```python
from build123d import *

# Parameters (mm, degrees)
F1_DEPTH = 295.5
F3_DEPTH = 50
F5_D     = 12.5


# Not quite as in the source:
# - a pattern or mirror of a feature is missing from the dataset's text; its kind, count and spacing are read off the source's solid


with BuildPart() as f1:
    # F0 (on Right) → F1 (new body, symmetric)
    with BuildSketch(Plane.YZ):
        Polygon((0, 6), (0, 0), (50, 0), (50, 50), (44, 50), (44, 6), align=None)
    extrude(amount=F1_DEPTH, both=True)

    # F2 (on face) → F3 (join)
    with BuildSketch(Plane(origin=(0, 50, 0), x_dir=(-1, 0, 0), z_dir=(0, 1, 0))):
        Polygon((-301.5, 0), (-295.5, 0), (-295.5, 50), (-345.5, 50), (-345.5, 44), (-301.5, 44), align=None)
    f3 = extrude(amount=-F3_DEPTH)

    # F3_copies: F3 across plane
    add(f3.mirror(Plane(origin=(0, 0, 0), x_dir=(0, 0, -1), z_dir=(-1, 0, 0))))

    # F5 (through all)
    with Locations(Plane.XY.offset(50)):
        with Locations((318, 37.5), (318, 12.5)):
            f5 = Hole(F5_D / 2)

    # F5_copies: F5 across plane
    add(f5.mirror(Plane(origin=(0, 0, 0), x_dir=(0, 0, -1), z_dir=(-1, 0, 0))), mode=Mode.SUBTRACT)


solid = f1.part
```
Geometry: final body of the model. Coordinates: model frame, mm. A direction names the side the tool comes from. Round coordinates to 2 decimals unless told otherwise and drop trailing zeros. Write each loop counter-clockwise with the first axis right and the second up, starting at its lowest first coordinate (ties: lowest second). Pieces come first, ordered by that corner, then holes. Notation, with made-up numbers: M 47.25,-0.75 L 86.25,-0.75 A21 cw 86.25,38.25 Z; hole C 55,8.25 d9. An arc over 180 degrees is marked long. Answer in a Markdown table with one row per item. Add a question column.
(1) Cut plane D-D, the plane x = 219. Return the cut outline in (y, z).
(2) Cut plane A-A, the plane x = -318. Return the cut outline in (y, z).
(3) Cut plane C-C, the plane z = 32. Return the cut outline in (x, y), then the cut area to 3 significant figures.
(4) Ray query, L1, parallel to Y at x = 318, z = 46; L2, parallel to X at y = 12, z = 47; L3, parallel to X at y = 14, z = 7.5. Return the intervals inside material, ascending.
(5) Cut plane B-B, the plane y = 37.5. Return the cut outline in (x, z), then the cut area to 3 significant figures.
(6) Draft query along X for faces 1 (the face through (324.244, 12.775, 46.958)), 2 (the face through (-4, 25, 0)), 3 (the face through (-301.5, 25, 22)), 4 (the face through (-324.244, 37.775, 46.958)). Return one class per face: pulls with the +X half, pulls with the -X half, needs draft (parallel to the pull), parting line crosses it, or undercut.
(7) Reachability of faces 5 (the face through (-2, 0, 5)), 6 (the face through (295.5, 22, 28)), 7 (the face through (-324, 25, 44)), 8 (the face through (301.5, 25, 22)), 9 (the face through (2, 45, 50)) from +Z, -Z, +X, -X, +Y, -Y: full face, straight path, thin tool, end or side. Return the list, or none.
(8) Contact query for flat-ended pins moving along their axis: pin 1 (4 mm diameter, centred on y = 33, z = 34.5, fed in from -X); pin 2 (12 mm diameter, centred on y = 10.5, z = 22.5, fed in from +X); pin 3 (3 mm diameter, centred on x = -84, y = 39, fed in from +Z); pin 4 (8 mm diameter, centred on x = -201, y = 25, fed in from -Z). Output: stop coordinate, or through.
Established:
| question | item | result |
|---|---|---|
| 1 | outline | M 0,0 L 50,0 L 50,50 L 44,50 L 44,6 L 0,6 Z |
| 2 | outline | M 0,44 L 6.25,44 L 6.25,50 L 0,50 Z; M 18.75,44 L 31.25,44 L 31.25,50 L 18.75,50 Z; M 43.75,44 L 50,44 L 50,50 L 43.75,50 Z |
| 3 | outline | M -301.5,0 L -295.5,0 L -295.5,44 L 295.5,44 L 295.5,0 L 301.5,0 L 301.5,50 L -301.5,50 Z |
| 3 | area | 4,150 mm² |
| 4 | L1 | 0 to 6.25, 18.75 to 31.25, 43.75 to 50 |
| 4 | L2 | -345.5 to -324.23, -311.77 to -295.5, 295.5 to 311.77, 324.23 to 345.5 |
| 4 | L3 | -301.5 to -295.5, 295.5 to 301.5 |
| 5 | outline | M -345.5,44 L -324.25,44 L -324.25,50 L -345.5,50 Z; M -311.75,44 L -301.5,44 L -301.5,0 L 301.5,0 L 301.5,44 L 311.75,44 L 311.75,50 L 295.5,50 L 295.5,6 L -295.5,6 L -295.5,50 L -311.75,50 Z; M 324.25,44 L 345.5,44 L 345.5,50 L 324.25,50 Z |
| 5 | area | 4,520 mm² |
| 6 | face 1 | undercut |
| 6 | face 2 | needs draft |
| 6 | face 3 | pulls with the -X half |
| 6 | face 4 | undercut |
| 7 | face 5 | +Z, -Z, +X, -X, -Y |
| 7 | face 6 | +Z, -Y |
| 7 | face 7 | -Z, -X, +Y, -Y |
| 7 | face 8 | -Z, +X, +Y, -Y |
| 7 | face 9 | +Z, +X, -X, +Y, -Y |
| 8 | pin 1 | x = -301.5 |
| 8 | pin 2 | x = 301.5 |
| 8 | pin 3 | z = 6 |
| 8 | pin 4 | z = 0 |
